Part print with two shaded views. Sizes in mm from the minimum x, y, z corner. A direction names the side the tool comes from. Give positions to 0.01 mm unless a question says otherwise; leave off trailing zeros. Write each loop counter-clockwise with the first axis right and the second up, starting at its lowest first coordinate (ties: lowest second). Pieces come first, ordered by that corner, then holes.
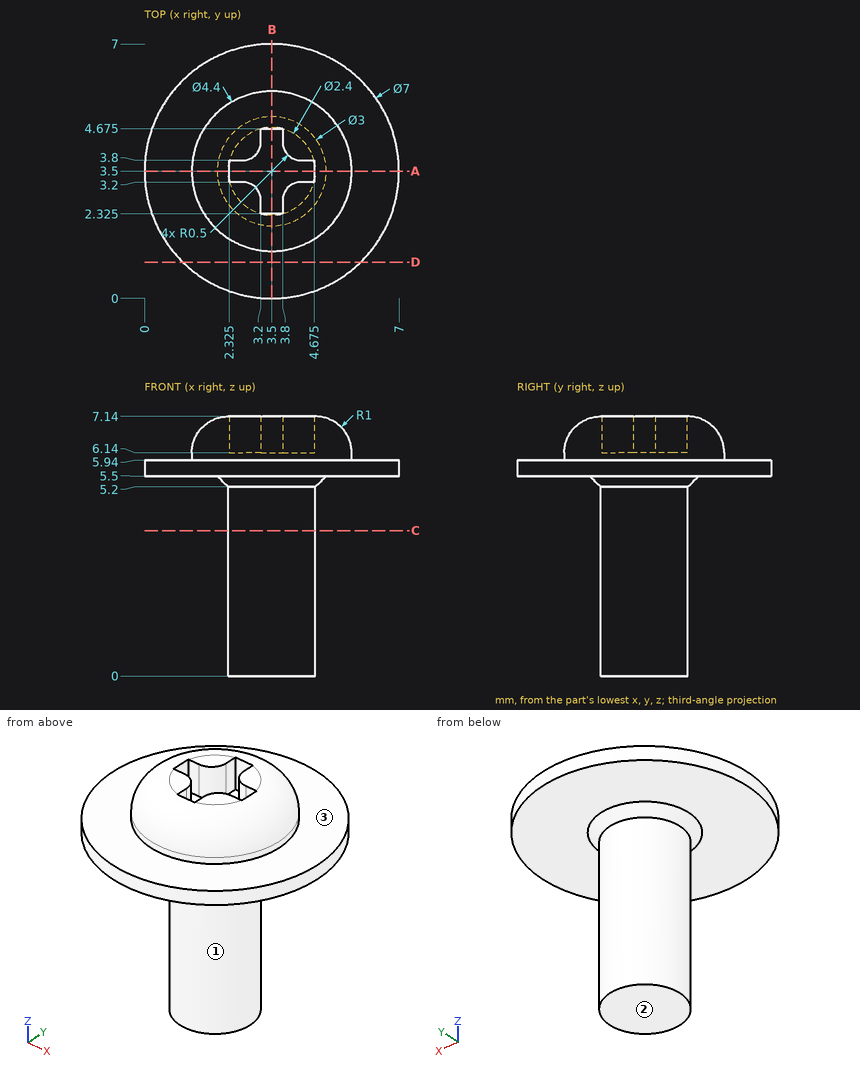
1) Pin check, flat tips, straight feed: pin 1 Ø1 at (y, z) = (2, 1) entering from +X; pin 2 Ø0.5 at (y, z) = (3.5, 7) entering from +X; pin 3 Ø3 at (y, z) = (5, 1.5) entering from +X; pin 4 Ø4 at (x, y) = (3.5, 4.5) entering from -Z. Stop position of each tip, or through.
Answers follow:
pin 1: stops at x = 4.16
pin 2: stops at x = 5.49
pin 3: stops at x = 4.7
pin 4: stops at z = 0
2) Saw through at C-C, the plane z = 4. Write the cut outline in (x, y).
Answers follow:
outline: circle Ø2.4 at (3.5, 3.5)
3) Wall check: L1, parallel to Z at x = 1, y = 1.5; L2, parallel to Y at x = 3.75, z = 4.25; L3, parallel to Y at x = 3.75, z = 7 (3 decimals). Give the ranges that are in metal, low to high.
Answers follow:
L1: z = 5.5 to 5.94
L2: y = 2.33 to 4.67
L3: y = 1.808 to 2.325, 4.675 to 5.192
4) Saw through at D-D, the plane y = 1. Write the cut outline in (x, z), then the cut area to 3 significant figures.
Answers follow:
outline: (1.05, 5.5) - (5.95, 5.5) - (5.95, 5.94) - (1.05, 5.94) - close
area: 2.16 mm2
5) 3-axis set-ups, long thin cutter, end or side, ignore diameter. For the marked faces 1, 2 and 3: which of +Z, -Z, +X, -X, +Y, -Y reach the whole face in a straight line?
Answers follow:
face 1: -Z
face 2: -Z, +X, -X, +Y, -Y
face 3: +Z
6) Saw through at A-A, the plane y = 3.5. Write the cut outline in (x, z) (3 decimals).
Answers follow:
outline: (0, 5.5) - (2, 5.5) - (2.3, 5.2) - (2.3, 0) - (4.7, 0) - (4.7, 5.2) - (5, 5.5) - (7, 5.5) - (7, 5.94) - (5.7, 5.94) - (5.7, 6.14) arc R1 ccw to (4.7, 7.14) - (4.675, 7.14) - (4.675, 6.14) - (2.325, 6.14) - (2.325, 7.14) - (2.3, 7.14) arc R1 ccw to (1.3, 6.14) - (1.3, 5.94) - (0, 5.94) - close
